Read the model definition and answer for the solid it produces. Units are mm, in the model's axes. Face numbers are marked on the shaded views. A direction names the side the tool comes from. Give positions to 0.01 mm unless a question says otherwise; leave off trailing zeros. Order: outer loops, then holes, each group sorted by start corner. A loop starts at its lowest first (then second) coordinate and runs counter-clockwise, first axis right, second up.
Item 1: Given pin 1 Ø1.8 at (x, y) = (22, 38.5) entering from -Z; pin 2 Ø5.5 at (x, y) = (-21.5, 37) entering from +Z; pin 3 Ø1 at (y, z) = (35, -37) entering from -X, each flat-ended and moving along its own axis, determine where each tip first touches the part or whether it passes through.
Item 2: A cutting plane is placed at D-D (z = -17.5). Write down the section's boundary in (x, y).
Item 3: Find the intervals of material crossed by line 1 along X through (y, z) = (58, -35); line 2 along Z through (x, y) = (20, 58.9); line 3 along Z through (x, y) = (5.5, 43.5), in increasing order.
Item 4: A cutting plane is placed at A-A (z = 0). Write down the section's boundary in (x, y).
Item 5: A cutting plane is placed at C-C (x = 12). Write down the section's boundary in (y, z), plus the area to 3 significant figures.
Item 6: The mould has two halves that part along X. Classify the marked faces 1, 2, 3 and 4: +X half, -X half, draft (parallel to the pull), parting line (faces both ways), or undercut.
Item 7: Which of the six approach directions +Z, -Z, +X, -X, +Y, -Y give full straight-line access (tool end or side, diameter ignored) to the marked faces 5, 6 and 7?
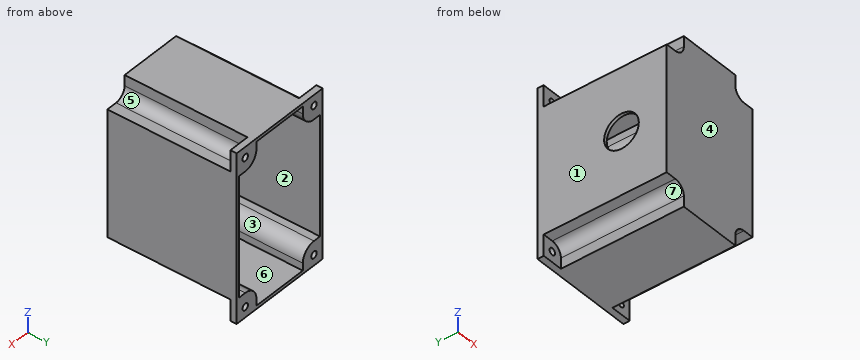
from build123d import *

# Parameters (mm, degrees)
BOSS_EXTRUDE6_DEPTH = 60
BOSS_EXTRUDE8_DEPTH = 1.5
BOSS_EXTRUDE9_DEPTH = 3
SKETCH15_R          = 1.6
CUT_EXTRUDE4_DEPTH  = 62.5
SKETCH11_R          = 8.25
CUT_EXTRUDE3_DEPTH  = 1.5


with BuildPart() as part:
    # Sketch1 → Boss-Extrude6 (new body)
    with BuildSketch(Plane(origin=(0, 0, 0), x_dir=(1, 0, 0), z_dir=(0, 1, 0))):
        with BuildLine():
            Line((-15, -35), (-15, -40))
            Line((-15, -40), (-13.5, -40))
            Line((-13.5, -40), (13.5, -40))
            Line((13.5, -40), (15, -40))
            Line((15, -40), (15, -35))
            ThreePointArc((15, -35), (16.464466094, -31.464466094), (20, -30))
            Line((20, -30), (25, -30))
            Line((25, -30), (25, -28.5))
            Line((25, -28.5), (25, 28.5))
            Line((25, 28.5), (25, 30))
            Line((25, 30), (20, 30))
            ThreePointArc((20, 30), (16.464466094, 31.464466094), (15, 35))
            Line((15, 35), (15, 40))
            Line((15, 40), (13.5, 40))
            Line((13.5, 40), (-13.5, 40))
            Line((-13.5, 40), (-15, 40))
            Line((-15, 40), (-15, 35))
            ThreePointArc((-15, 35), (-16.464466094, 31.464466094), (-20, 30))
            Line((-20, 30), (-25, 30))
            Line((-25, 30), (-25, 28.5))
            Line((-25, 28.5), (-25, -28.5))
            Line((-25, -28.5), (-25, -30))
            Line((-25, -30), (-20, -30))
            ThreePointArc((-20, -30), (-16.464466094, -31.464466094), (-15, -35))
        make_face()
        with BuildLine():
            Line((20, 28.5), (23.5, 28.5))
            Line((23.5, 28.5), (23.5, -28.5))
            Line((23.5, -28.5), (20, -28.5))
            ThreePointArc((20, -28.5), (15.403805922, -30.403805922), (13.5, -35))
            Line((13.5, -35), (13.5, -38.5))
            Line((13.5, -38.5), (-13.5, -38.5))
            Line((-13.5, -38.5), (-13.5, -35))
            ThreePointArc((-13.5, -35), (-15.403805922, -30.403805922), (-20, -28.5))
            Line((-20, -28.5), (-23.5, -28.5))
            Line((-23.5, -28.5), (-23.5, 28.5))
            Line((-23.5, 28.5), (-20, 28.5))
            ThreePointArc((-20, 28.5), (-15.403805922, 30.403805922), (-13.5, 35))
            Line((-13.5, 35), (-13.5, 38.45))
            Line((-13.5, 38.45), (13.5, 38.45))
            Line((13.5, 38.45), (13.5, 35))
            ThreePointArc((13.5, 35), (15.403805922, 30.403805922), (20, 28.5))
        make_face(mode=Mode.SUBTRACT)
    extrude(amount=BOSS_EXTRUDE6_DEPTH)

    # Sketch7 → Boss-Extrude8 (add)
    with BuildSketch(Plane.XZ):
        with BuildLine():
            Line((-15, 40), (15, 40))
            Line((15, 40), (15, 35))
            ThreePointArc((15, 35), (16.464466094, 31.464466094), (20, 30))
            Line((20, 30), (25, 30))
            Line((25, 30), (25, -30))
            Line((25, -30), (20, -30))
            ThreePointArc((20, -30), (16.464466094, -31.464466094), (15, -35))
            Line((15, -35), (15, -40))
            Line((15, -40), (-15, -40))
            Line((-15, -40), (-15, -35))
            ThreePointArc((-15, -35), (-16.464466094, -31.464466094), (-20, -30))
            Line((-20, -30), (-25, -30))
            Line((-25, -30), (-25, 30))
            Line((-25, 30), (-20, 30))
            ThreePointArc((-20, 30), (-16.464466094, 31.464466094), (-15, 35))
            Line((-15, 35), (-15, 40))
        make_face()
    extrude(amount=BOSS_EXTRUDE8_DEPTH)

    # Sketch12 → Boss-Extrude9 (add)
    with BuildSketch(Plane(origin=(0, 60, 0), x_dir=(1, 0, 0), z_dir=(0, 1, 0))):
        with BuildLine():
            Line((-25, 40), (-15, 40))
            Line((-15, 40), (-15, 35))
            ThreePointArc((-15, 35), (-16.464466094, 31.464466094), (-20, 30))
            Line((-20, 30), (-25, 30))
            Line((-25, 30), (-25, 40))
        make_face()
        with BuildLine():
            Line((15, 40), (25, 40))
            Line((25, 40), (25, 30))
            Line((25, 30), (20, 30))
            ThreePointArc((20, 30), (16.464466094, 31.464466094), (15, 35))
            Line((15, 35), (15, 40))
        make_face()
        with BuildLine():
            Line((20, -30), (25, -30))
            Line((25, -30), (25, -40))
            Line((25, -40), (15, -40))
            Line((15, -40), (15, -35))
            ThreePointArc((15, -35), (16.464466094, -31.464466094), (20, -30))
        make_face()
        with BuildLine():
            Line((-15, -40), (-25, -40))
            Line((-25, -40), (-25, -30))
            Line((-25, -30), (-20, -30))
            ThreePointArc((-20, -30), (-16.464466094, -31.464466094), (-15, -35))
            Line((-15, -35), (-15, -40))
        make_face()
    extrude(amount=-BOSS_EXTRUDE9_DEPTH)

    # Sketch15 → Cut-Extrude4 (cut, through all)
    with BuildSketch(Plane(origin=(0, 60, 0), x_dir=(1, 0, 0), z_dir=(0, 1, 0))):
        with Locations((-20, -35)):
            Circle(SKETCH15_R)
        with Locations((20, -35)):
            Circle(SKETCH15_R)
        with Locations((20, 35)):
            Circle(SKETCH15_R)
        with Locations((-20, 35)):
            Circle(SKETCH15_R)
    extrude(amount=-CUT_EXTRUDE4_DEPTH, mode=Mode.SUBTRACT)

    # Sketch11 → Cut-Extrude3 (cut)
    with BuildSketch(Plane.ZY.offset(25)):
        with Locations((0, 20)):
            Circle(SKETCH11_R)
    extrude(amount=-CUT_EXTRUDE3_DEPTH, mode=Mode.SUBTRACT)


solid = part.part
Response values:
1. pin 1: stops at z = -30
1. pin 2: stops at z = 30.16
1. pin 3: stops at x = -15
2. outline: (-25, -1.5) - (25, -1.5) - (25, 60) - (23.5, 60) - (23.5, 0) - (-23.5, 0) - (-23.5, 60) - (-25, 60) - close
3. line 1: x = -25 to -21.6, -18.4 to -13.5, 13.5 to 18.4, 21.6 to 25
3. line 2: z = -40 to -36.6, -33.4 to -28.5, 28.5 to 33.4, 36.6 to 40
3. line 3: z = -40 to -38.45, 38.5 to 40
4. outline: (-25, -1.5) - (25, -1.5) - (25, 60) - (23.5, 60) - (23.5, 0) - (-23.5, 0) - (-23.5, 11.75) - (-25, 11.75) - close; (-25, 28.25) - (-23.5, 28.25) - (-23.5, 60) - (-25, 60) - close
5. outline: (-1.5, -40) - (60, -40) - (60, -38.45) - (0, -38.45) - (0, 38.5) - (60, 38.5) - (60, 40) - (-1.5, 40) - close
5. area: 303 mm2
6. face 1: -X half
6. face 2: undercut
6. face 3: undercut
6. face 4: draft
7. face 5: +Z, +X, -Y
7. face 6: +Y
7. face 7: -Z, -X, -Y
